```python
from build123d import *

# Parameters (mm, degrees)
F1_DEPTH = 15
F2_R     = 1.7
F3_DEPTH = 28.8924828911
F5_DEPTH = 1.38
F6_R     = 4.99999


# Not quite as in the source:
# - a fillet or chamfer is up to 0.001 mm smaller than in the source, because OpenCascade refuses the exact size


with BuildPart() as f1:
    # F0 (on Top) → F1 (new body)
    with BuildSketch(Plane.XY):
        Polygon((9.275, 35), (9.275, -35), (-9.275, -35), (-9.275, 35), (-14.275, 35), (-14.275, -35), (-14.275, -45), (59.6164828911, -45), (59.6164828911, -35), (54.6164828911, -25), (54.6164828911, -35), (14.6164828911, -35), (14.6164828911, 35), align=None)
    extrude(amount=F1_DEPTH)

    # F2 (on face) → F3 (cut, through all)
    with BuildSketch(Plane.YZ.offset(14.6164828911)):
        with Locations((0, 7.5)):
            Circle(F2_R)
    extrude(amount=-F3_DEPTH, mode=Mode.SUBTRACT)

    # F4 (on face) → F5 (cut)
    with BuildSketch(Plane(origin=(-14.275, 0, 0), x_dir=(0, -1, 0), z_dir=(-1, 0, 0))):
        Polygon((-2.2689865579, 3.57), (2.2689865579, 3.57), (4.5379731158, 7.5), (2.2689865579, 11.43), (-2.2689865579, 11.43), (-4.5379731158, 7.5), align=None)
    extrude(amount=-F5_DEPTH, mode=Mode.SUBTRACT)

    # F6 (radius 5 in the source; OpenCascade refuses exactly that, so slightly less here)
    f6_edges = [f1.edges().sort_by_distance(p)[0] for p in [
        (-9.275, -35, 7.5),
        (9.275, -35, 7.5),
        (-14.275, -45, 7.5),
        (59.616483, -45, 7.5),
        (54.616483, -35, 7.5),
        (14.616483, -35, 7.5),
        (59.616483, -35, 7.5),
        (14.616483, 35, 7.5),
        (-14.275, 35, 7.5),
    ]]
    fillet(f6_edges, radius=F6_R)


solid = f1.part
```
Can you work these out from the model? Positions are in its coordinate system, mm. A direction names the side the tool comes from. Round coordinates to 2 decimals unless told otherwise and drop trailing zeros. Loops run counter-clockwise (first coordinate to the right, second up) from the corner with the lowest first, then second, coordinate; pieces in that order, holes last. Notation, with made-up numbers: M -30,28.5 L -6,28.5 A33 ccw -6,57.5 Z; hole C 87,6.5 d11. An arc over 180 degrees is marked long. Write item = value, one per line. Start each with the question number.
(1) Suppose I cut it at D-D on y = -31. Write out the boundary of the cut face in (x, z) (1 decimal), plus the area to 3 significant figures.
(2) If we mould it in two halves opening along X, with no side actions, what happens to faces 1 (the face through (54.616, -27, 7)), 2 (the face through (-14.275, -5, 7)), 3 (the face through (12, -20, 15))? For each: released by +X, released by -X, zero draft, split by the parting line, or undercut.
(3) Suppose I cut it at B-B on y = 0. Write out the boundary of the cut face in (x, z) (3 decimals), plus the area to 3 significant figures.
(4) I need wall thicknesses on line 1 along X through (y, z) = (13, 7.25) (3 decimals); line 2 along Z through (x, y) = (-10, 0); line 3 along Y through (x, z) = (2, 7.5). Which ranges of each line are inside material? Lowest first, please.
(5) Which directions (+Z, -Z, +X, -X, +Y, -Y) give clear straight access to the entire face, cutting with the end or side of a thin tool? Please do faces 4 (the face through (56.88, -29.53, 7.4)), 5 (the face through (-13.59, 3.39, 9.49)), 6 (the face through (-9.275, 2, 7)).
(6) I'm going to push flat-ended pins straight in: P1, Ø2, axis at y = -28, z = 13.5, coming from the +X side; P2, Ø4.5, axis at y = 2.5, z = 4.5, coming from the +X side; P3, Ø4.5, axis at x = 1.5, z = 8.5, coming from the +Y side. Where does each tip first touch, or does it pass through?
(7) Suppose I cut it at A-A on y = 23.5. Write out the boundary of the cut face in (x, z) (3 decimals).
Answer block:
q1.outline = M -14.3,0 L -9.2,0 L -9.2,15 L -14.3,15 Z; M 9.2,0 L 14.7,0 L 14.7,15 L 9.2,15 Z; M 54.5,0 L 57.6,0 L 57.6,15 L 54.5,15 Z
q1.area = 206 mm²
q2.face_1 = undercut
q2.face_2 = released by -X
q2.face_3 = zero draft
q3.outline = M -14.275,0 L -9.275,0 L -9.275,5.8 L -12.895,5.8 L -12.895,3.57 L -14.275,3.57 Z; M -14.275,11.43 L -12.895,11.43 L -12.895,9.2 L -9.275,9.2 L -9.275,15 L -14.275,15 Z; M 9.275,0 L 14.616,0 L 14.616,5.8 L 9.275,5.8 Z; M 9.275,9.2 L 14.616,9.2 L 14.616,15 L 9.275,15 Z
q3.area = 114 mm²
q4.line_1 = -14.275 to -9.275, 9.275 to 14.616
q4.line_2 = 0 to 5.8, 9.2 to 15
q4.line_3 = -45 to -35
q5.face_4 = +Z, -Z, +X, +Y
q5.face_5 = -X
q5.face_6 = +Z, -Z, +Y
q6.P1 = 56.62
q6.P2 = 14.62
q6.P3 = -35
q7.outline = M -14.275,0 L -9.275,0 L -9.275,15 L -14.275,15 Z; M 9.275,0 L 14.616,0 L 14.616,15 L 9.275,15 Z
